```python
from build123d import *

# Parameters (mm, degrees)
SALIENTE_EXTRUIR1_DEPTH = 65
CROQUIS2_R              = 4.7625
CORTAR_EXTRUIR1_DEPTH   = 130
CROQUIS3_R              = 6.5
CORTAR_EXTRUIR2_DEPTH   = 130


with BuildPart() as part:
    # Croquis1 → Saliente-Extruir1 (new, symmetric)
    with BuildSketch(Plane.XY):
        Polygon((0, 0), (0, 480), (-4.7625, 480), (-4.7625, 4.7625), (-70, 4.7625), (-70, 0), align=None)
    extrude(amount=SALIENTE_EXTRUIR1_DEPTH, both=True)

    # Croquis2 → Cortar-Extruir1 (cut)
    with BuildSketch(Plane(origin=(0, 0, 0), x_dir=(-1, 0, 0), z_dir=(0, -1, 0))):
        with Locations(Location((35, -32.5, 0), (0, 0, 180))):
            Circle(CROQUIS2_R)
        with Locations(Location((35, 32.5, 0), (0, 0, 180))):
            Circle(CROQUIS2_R)
    extrude(amount=-CORTAR_EXTRUIR1_DEPTH, mode=Mode.SUBTRACT)

    # Croquis3 → Cortar-Extruir2 (cut)
    with BuildSketch(Plane(origin=(0, 0, 0), x_dir=(0, 0, -1), z_dir=(1, 0, 0))):
        with Locations((-34.13125, 455)):
            Circle(CROQUIS3_R)
        with Locations((34.13125, 455)):
            Circle(CROQUIS3_R)
    extrude(amount=-CORTAR_EXTRUIR2_DEPTH, mode=Mode.SUBTRACT)


solid = part.part
```
Geometry check sheet. Reference: the model listing, model coordinates, mm. A direction names the side the tool comes from. Coordinates: 2 decimals unless noted, no trailing zeros. Loops run counter-clockwise (first coordinate to the right, second up) from the corner with the lowest first, then second, coordinate; pieces in that order, holes last. Notation, with made-up numbers: (66, 57) - (86, 57) arc R33 cw to (86, 87) - close; hole circle Ø11 at (78, 11.25). An arc over 180 degrees is marked (long way). One line per item, written item: value. Start each with the question number.
(1) Cross-section at D-D on z = -45.5. Enter the section's corners in (x, y), plus the area to 3 significant figures.
(2) Tool access check on faces 1 (the flat face through (-37, 4.762, 1)), 2 (the cylindrical face through (-2.348, 461.445, 34.977)). Record the directions out of +Z, -Z, +X, -X, +Y, -Y that give a thin tool (end or side, any length) a straight path to the whole face; none if there is none.
(3) Cross-section at B-B on x = -35. Enter the section's corners in (y, z).
(4) Mould release check, pull along Z, two halves, no side actions. Record for faces 3 (the flat face through (-1, 241, -65)), 4 (the flat face through (-1, 241, 65)), 5 (the cylindrical face through (-35.62, 2.35, -27.78)), 6 (the flat face through (0, 237, 1)): released by +Z, released by -Z, zero draft, split by the parting line, or undercut.
(5) Cross-section at C-C on z = 32.5. Enter the section's corners in (x, y), plus the area to 3 significant figures.
(6) Depth check by flat-ended pin: P1, Ø1.5, axis at y = 387.5, z = -11, coming from the -X side. Enter the tip coordinate at first touch or a pass-through.
(7) Material ranges on line 1 (Z direction, x = -2, y = 455); line 2 (Y direction, x = -40.5, z = 47); line 3 (X direction, y = 394, z = 37), recorded low to high. Write a range as [from, to].
(8) Cross-section at A-A on y = 455. Enter the section's corners in (x, z).
Results below:
1. outline: (-70, 0) - (0, 0) - (0, 480) - (-4.76, 480) - (-4.76, 4.76) - (-70, 4.76) - close
1. area: 2,600 mm2
2. face 1: +Z, -Z, -X, +Y
2. face 2: +X, -X
3. outline: (0, -65) - (4.76, -65) - (4.76, -37.26) - (0, -37.26) - close; (0, -27.74) - (4.76, -27.74) - (4.76, 27.74) - (0, 27.74) - close; (0, 37.26) - (4.76, 37.26) - (4.76, 65) - (0, 65) - close
4. face 3: released by -Z
4. face 4: released by +Z
4. face 5: undercut
4. face 6: zero draft
5. outline: (-70, 0) - (-39.76, 0) - (-39.76, 4.76) - (-70, 4.76) - close; (-30.24, 0) - (0, 0) - (0, 448.71) - (-4.76, 448.71) - (-4.76, 4.76) - (-30.24, 4.76) - close; (-4.76, 461.29) - (0, 461.29) - (0, 480) - (-4.76, 480) - close
5. area: 2,490 mm2
6. P1: stops at x = -4.76
7. line 1: z = [-65, -40.63], [-27.63, 27.63], [40.63, 65]
7. line 2: y = [0, 4.76]
7. line 3: x = [-4.76, 0]
8. outline: (-4.76, -65) - (0, -65) - (0, -40.63) - (-4.76, -40.63) - close; (-4.76, -27.63) - (0, -27.63) - (0, 27.63) - (-4.76, 27.63) - close; (-4.76, 40.63) - (0, 40.63) - (0, 65) - (-4.76, 65) - close
